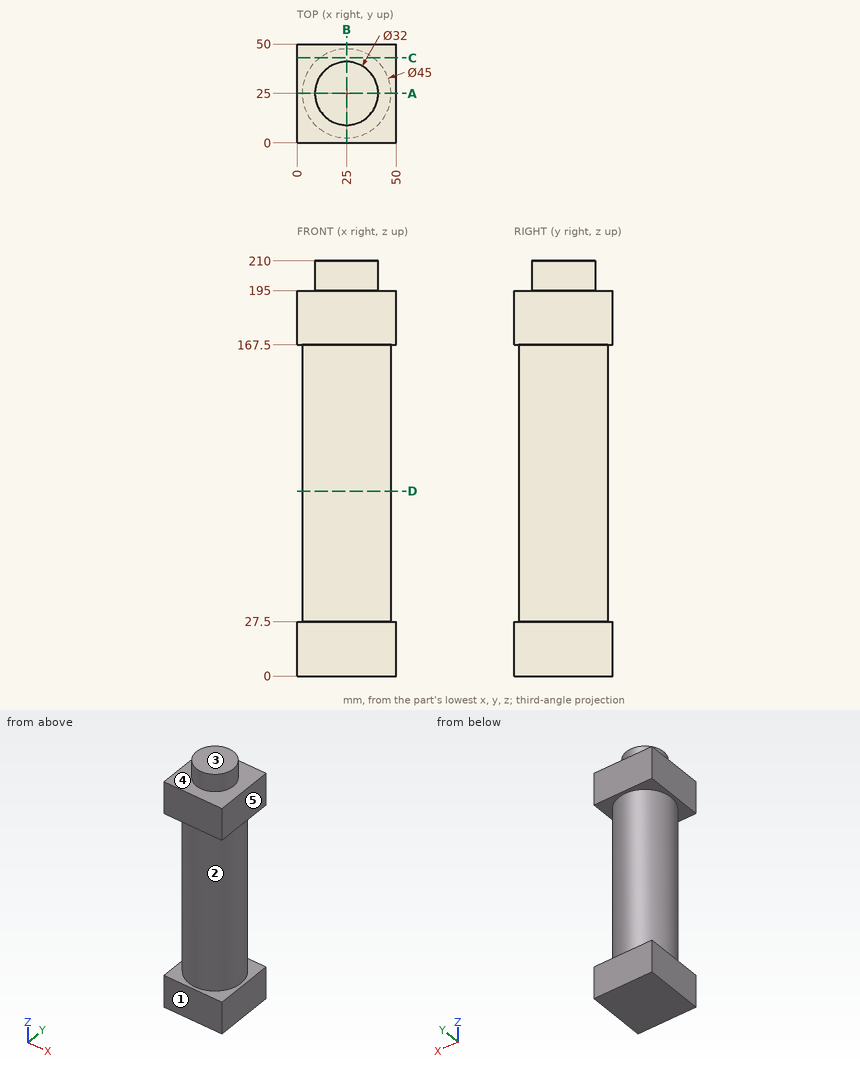
Answer from the drawing. Dimensions are ordinates in mm from the lowest x, y and z of the part. A direction names the side the tool comes from. Give positions to 0.01 mm unless a question says otherwise; leave off trailing zeros. Write each loop counter-clockwise with the first axis right and the second up, starting at its lowest first coordinate (ties: lowest second). Pieces come first, ordered by that corner, then holes. Notation, with made-up numbers: M -30,50.5 L -20,50.5 A22 cw -20,57.5 Z; hole C 13.5,-23 d9. An arc over 180 degrees is marked long. Answer as CSV lines item,"result".
Q1. The mould has two halves that part along Z. Classify the marked faces 1, 2 and 3: +Z half, -Z half, draft (parallel to the pull), parting line (faces both ways), or undercut.
A:
face 1,"draft"
face 2,"undercut"
face 3,"+Z half"
Q2. Given P1, Ø10, axis at x = 21.5, z = 55.5, coming from the +Y side; P2, Ø6, axis at y = 16.5, z = 71, coming from the -X side; P3, Ø1.5, axis at x = 35.5, z = 113, coming from the +Y side, each flat-ended and moving along its own axis, determine where each tip first touches the part or whether it passes through.
A:
P1,"stops at y = 47.5"
P2,"stops at x = 3.18"
P3,"stops at y = 45.28"
Q3. A cutting plane is placed at C-C on y = 43. Write down the section's boundary in (x, z).
A:
outline,"M 0,0 L 50,0 L 50,27.5 L 38.5,27.5 L 38.5,167.5 L 50,167.5 L 50,195 L 0,195 L 0,167.5 L 11.5,167.5 L 11.5,27.5 L 0,27.5 Z"
Q4. Find the intervals of material crossed by probe 1 along Z at (x, y) = (45, 43); probe 2 along Y at (x, z) = (24, 116); probe 3 along X at (y, z) = (25.5, 126), in increasing order. Write a range as [from, to].
A:
probe 1,"z = [0, 27.5], [167.5, 195]"
probe 2,"y = [2.52, 47.48]"
probe 3,"x = [2.51, 47.49]"
Q5. A tool of negligible diameter and unlimited length cuts with its end or side. For the marked faces 4 and 5, from which of +Z, -Z, +X, -X, +Y, -Y can it reach the whole face along a straight path? Write none if from no direction.
A:
face 4,"+Z"
face 5,"+Z, -Z, +X, +Y, -Y"
Q6. A cutting plane is placed at A-A on y = 25. Write down the section's boundary in (x, z).
A:
outline,"M 0,0 L 50,0 L 50,27.5 L 47.5,27.5 L 47.5,167.5 L 50,167.5 L 50,195 L 41,195 L 41,210 L 9,210 L 9,195 L 0,195 L 0,167.5 L 2.5,167.5 L 2.5,27.5 L 0,27.5 Z"
Q7. A cutting plane is placed at D-D on z = 93.5. Write down the section's boundary in (x, y).
A:
outline,"C 25,25 d45"
